```python
from build123d import *

# Parameters (mm, degrees)
BOSS_EXTRUDE1_DEPTH   = 349
M4_CLEARANCE_HOLE1_D  = 4.5
M4X0_7_TAPPED_HOLE1_D = 3.3


with BuildPart() as part:
    # Sketch1 → Boss-Extrude1 (new body)
    with BuildSketch(Plane.XY):
        Polygon((0, 0), (12.7, 0), (12.7, -1.524), (1.524, -1.524), (1.524, -12.7), (0, -12.7), align=None)
    extrude(amount=BOSS_EXTRUDE1_DEPTH)

    # M4 Clearance Hole1 (through all)
    with Locations(Plane(origin=(0, 0, 0), x_dir=(1, 0, 0), z_dir=(0, 1, 0))):
        with Locations((6.35, -7), (6.35, -342)):
            Hole(M4_CLEARANCE_HOLE1_D / 2)

    # M4x0.7 Tapped Hole1 (through all)
    with Locations(Plane.ZY):
        with Locations((65.553973, -6.35), (283.446027, -6.35)):
            Hole(M4X0_7_TAPPED_HOLE1_D / 2)


solid = part.part
```
Part model, mm, in its own coordinate system. A direction names the side the tool comes from. Give positions to 0.01 mm unless a question says otherwise; leave off trailing zeros. Write each loop counter-clockwise with the first axis right and the second up, starting at its lowest first coordinate (ties: lowest second). Pieces come first, ordered by that corner, then holes. Notation, with made-up numbers: (45.5, 68.25) -> (68.5, 68.25) arc R19 cw to (68.5, 103.25) -> close; hole circle Ø7 at (32, 22.5). An arc over 180 degrees is marked (long way). Put each result on its own line as item: value. Start each with the question number.
Item 1: Which spindle directions (+Z, -Z, +X, -X, +Y, -Y) get a long thin tool onto all of the face, cutting with end or side? Do faces 1 (the face through (4, -1, 0)), 2 (the face through (1.524, -7, 172)). Say none if no direction does.
Item 2: Cut at C-C (y = -10.25). List the corners of the cut face in (x, z).
Item 3: Pin check, flat tip, straight feed: pin 1 Ø4 at (y, z) = (-6.35, 65.55) entering from +X. Stop position of the tip, or through.
Item 4: Cut at B-B (z = 175.5). List the corners of the cut face in (x, y).
Item 5: Wall check: L1, parallel to Z at x = 6.35, y = -0.5; L2, parallel to X at y = -0.25, z = 342; L3, parallel to X at y = -10.75, z = 100. Give the ranges that are in metal, low to high. Write a range as [from, to].
Item 6: Cut at A-A (x = 6.35). List the corners of the cut face in (y, z).
Answer list:
1. face 1: -Z, +X, -X, +Y, -Y
1. face 2: +Z, -Z, +X, -Y
2. outline: (0, 0) -> (1.52, 0) -> (1.52, 349) -> (0, 349) -> close
3. pin 1: stops at x = 1.52
4. outline: (0, -12.7) -> (1.52, -12.7) -> (1.52, -1.52) -> (12.7, -1.52) -> (12.7, 0) -> (0, 0) -> close
5. L1: z = [0, 4.75], [9.25, 339.75], [344.25, 349]
5. L2: x = [0, 4.1], [8.6, 12.7]
5. L3: x = [0, 1.52]
6. outline: (-1.52, 0) -> (0, 0) -> (0, 4.75) -> (-1.52, 4.75) -> close; (-1.52, 9.25) -> (0, 9.25) -> (0, 339.75) -> (-1.52, 339.75) -> close; (-1.52, 344.25) -> (0, 344.25) -> (0, 349) -> (-1.52, 349) -> close
